Work out the finished part from the listing and answer in its coordinate system (mm). A direction names the side the tool comes from. Give positions to 0.01 mm unless a question says otherwise; leave off trailing zeros. Order: outer loops, then holes, each group sorted by start corner. A loop starts at its lowest first (then second) coordinate and runs counter-clockwise, first axis right, second up.
```python
from build123d import *

# Parameters (mm, degrees)
F0_R          = 12.7
F1_DEPTH      = 12.7
F2_R          = 31.75
F3_DEPTH      = 5.08
F4_R          = 4.318
F5_DEPTH      = 12.701
F5_DEPTH_BACK = 95


# Not quite as in the source:
# - an extrude ends at something that could not be found from the text; its depth is read off the source's solid


with BuildPart() as f1:
    # F0 (on Front) → F1 (new body)
    with BuildSketch(Plane.XZ):
        Circle(F0_R)
    extrude(amount=F1_DEPTH)

    # F2 (on Front) → F3 (join)
    with BuildSketch(Plane.XZ):
        Circle(F2_R)
    extrude(amount=F3_DEPTH)

    # F4 (on Front) → F5 (cut, two sides)
    with BuildSketch(Plane.XZ) as f5_sk:
        Circle(F4_R)
    extrude(amount=F5_DEPTH, mode=Mode.SUBTRACT)
    extrude(f5_sk.sketch, amount=-F5_DEPTH_BACK, mode=Mode.SUBTRACT)


solid = f1.part
```
1. Given P1, Ø5, axis at x = -9, z = 18, coming from the -Y side; P2, Ø1, axis at x = -24.5, y = -1.5, coming from the -Z side; P3, Ø3, axis at y = -4.5, z = -19, coming from the -X side, each flat-ended and moving along its own axis, determine where each tip first touches the part or whether it passes through.
Findings below:
P1: stops at y = -5.08
P2: stops at z = -20.79
P3: stops at x = -26.49
2. Which of the six approach directions +Z, -Z, +X, -X, +Y, -Y give full straight-line access (tool end or side, diameter ignored) to faces 1 (the face through (5, -12.7, 0)), 2 (the face through (-2.75, -8.84, -12.4))?
Findings below:
face 1: +Z, -Z, +X, -X, -Y
face 2: -Y
3. The part is cut by section D-D (x = -11.5). Write down the section's boundary in (y, z), then the cut area to 3 significant figures.
Findings below:
outline: (-12.7, -5.39) - (-5.08, -5.39) - (-5.08, -29.59) - (0, -29.59) - (0, 29.59) - (-5.08, 29.59) - (-5.08, 5.39) - (-12.7, 5.39) - close
area: 383 mm2
4. The mould has two halves that part along Z. Classify faces 3 (the face through (-6.883, -2.504, -30.995)), 4 (the face through (7, 0, 0)), 5 (the face through (-0.56, -6.26, 4.28)): pulls with the +Z half, pulls with the -Z half, needs draft (parallel to the pull), parting line crosses it, or undercut.
Findings below:
face 3: parting line crosses it
face 4: needs draft
face 5: undercut
5. Straight lines are drawn through the part: probe 1 along Z at (x, y) = (0, -4.5); probe 2 along Z at (x, y) = (0, -8.75). For each, find the intervals that lie inside material, in ascending order.
Findings below:
probe 1: z = -31.75 to -4.32, 4.32 to 31.75
probe 2: z = -12.7 to -4.32, 4.32 to 12.7
6. The part is cut by section B-B (x = 0). Write down the section's boundary in (y, z), then the cut area to 3 significant figures.
Findings below:
outline: (-12.7, -12.7) - (-5.08, -12.7) - (-5.08, -31.75) - (0, -31.75) - (0, -4.32) - (-12.7, -4.32) - close; (-12.7, 4.32) - (0, 4.32) - (0, 31.75) - (-5.08, 31.75) - (-5.08, 12.7) - (-12.7, 12.7) - close
area: 406 mm2
7. The part is cut by section A-A (z = 0). Write down the section's boundary in (x, y).
Findings below:
outline: (-31.75, -5.08) - (-12.7, -5.08) - (-12.7, -12.7) - (-4.32, -12.7) - (-4.32, 0) - (-31.75, 0) - close; (4.32, -12.7) - (12.7, -12.7) - (12.7, -5.08) - (31.75, -5.08) - (31.75, 0) - (4.32, 0) - close
8. The part is cut by section C-C (y = -8.5). Write down the section's boundary in (x, z).
Findings below:
outline: circle Ø25.4 at (0, 0); hole circle Ø8.64 at (0, 0)
